Can you work these out from the model? Positions are in its coordinate system, mm. Round coordinates to 2 decimals unless told otherwise and drop trailing zeros. Order: outer loops, then holes, each group sorted by start corner. A loop starts at its lowest first (then second) coordinate and runs counter-clockwise, first axis right, second up. Notation, with made-up numbers: M -9.5,-8.5 L 13.5,-8.5 A17 ccw 13.5,-1.5 Z; hole C 20.5,-32.75 d1. An arc over 180 degrees is marked long. Answer as a JSON object with one key per item and string values. Group by question number.
from build123d import *

# Parameters (mm, degrees)
SKETCH_1_W      = 28
SKETCH_1_H      = 5
SKETCH_1_R      = 1.35
EXTRUDE_1_DEPTH = 2
FILLET_1_R      = 2


with BuildPart() as part:
    # 草图1 → 凸台-拉伸1 (new body)
    with BuildSketch(Plane.XY):
        Rectangle(SKETCH_1_W, SKETCH_1_H)
        with Locations((-11.5, 0)):
            Circle(SKETCH_1_R, mode=Mode.SUBTRACT)
        with Locations(Location((11.5, 0, 0), (0, 0, 180))):
            Circle(SKETCH_1_R, mode=Mode.SUBTRACT)
        Circle(SKETCH_1_R, mode=Mode.SUBTRACT)
    extrude(amount=EXTRUDE_1_DEPTH)

    # 圆角1
    fillet_1_edges = [part.edges().sort_by_distance(p)[0] for p in [
        (14, -2.5, 1),
        (-14, -2.5, 1),
        (-14, 2.5, 1),
        (14, 2.5, 1),
    ]]
    fillet(fillet_1_edges, radius=FILLET_1_R)


solid = part.part
Item 1: If we mould it in two halves opening along Y, with no side actions, what happens to faces 1 (the face through (0, 2, 2)), 2 (the face through (0, -2.5, 1)), 3 (the face through (-0.29, -1.32, 0.99))? For each: +Y half, -Y half, draft (parallel to the pull), parting line (faces both ways), or undercut.
Item 2: Suppose I cut it at C-C, the plane y = -1. Write out the boundary of the cut face in (x, z).
Item 3: Suppose I cut it at A-A, the plane x = -11.5. Write out the boundary of the cut face in (y, z), and give its area (3 significant figures).
Item 4: I need wall thicknesses on line 1 (Y direction, x = -11.5, z = 1); line 2 (X direction, y = 0.95, z = 1.55); line 3 (X direction, y = 0.85, z = 1.1). Which ranges of each line are inside material? Lowest first, please.
Item 5: Suppose I cut it at B-B, the plane z = 1. Write out the boundary of the cut face in (x, y).
Item 6: Suppose I cut it at D-D, the plane x = -0.5. Write out the boundary of the cut face in (y, z), and give its area (3 significant figures).
Computed:
{
 "1": {"face 1": "draft", "face 2": "-Y half", "face 3": "undercut"},
 "2": {"outline": "M -13.94,0 L -12.41,0 L -12.41,2 L -13.94,2 Z; M -10.59,0 L -0.91,0 L -0.91,2 L -10.59,2 Z; M 0.91,0 L 10.59,0 L 10.59,2 L 0.91,2 Z; M 12.41,0 L 13.94,0 L 13.94,2 L 12.41,2 Z"},
 "3": {"outline": "M -2.5,0 L -1.35,0 L -1.35,2 L -2.5,2 Z; M 1.35,0 L 2.5,0 L 2.5,2 L 1.35,2 Z", "area": "4.60 mm^2"},
 "4": {"line 1": "y = -2.5 to -1.35, 1.35 to 2.5", "line 2": "x = -13.95 to -12.46, -10.54 to -0.96, 0.96 to 10.54, 12.46 to 13.95", "line 3": "x = -13.97 to -12.55, -10.45 to -1.05, 1.05 to 10.45, 12.55 to 13.97"},
 "5": {"outline": "M -14,-0.5 A2 ccw -12,-2.5 L 12,-2.5 A2 ccw 14,-0.5 L 14,0.5 A2 ccw 12,2.5 L -12,2.5 A2 ccw -14,0.5 Z; hole C -11.5,0 d2.7; hole C 0,0 d2.7; hole C 11.5,0 d2.7"},
 "6": {"outline": "M -2.5,0 L -1.25,0 L -1.25,2 L -2.5,2 Z; M 1.25,0 L 2.5,0 L 2.5,2 L 1.25,2 Z", "area": "4.98 mm^2"}
}
